```python
from build123d import *

# Parameters (mm, degrees)
SKETCH_1_R      = 1.6
SKETCH_1_R_2    = 20.5
SKETCH_1_R_3    = 12.6
EXTRUDE_1_DEPTH = 2
FILLET_1_R      = 5


with BuildPart() as part:
    # 草图1 → 凸台-拉伸1 (new body)
    # profile 1 of 2: a face of its own
    with BuildSketch(Plane(origin=(0, 0, 0), x_dir=(1, 0, 0), z_dir=(0, 1, 0))):
        with BuildLine():
            Line((-20.5, 39.5), (-20.5, 0))
            ThreePointArc((-20.5, 0), (0, 20.5), (20.5, 0))
            Line((20.5, 0), (20.5, 39.5))
            Line((20.5, 39.5), (-20.5, 39.5))
        make_face()
        with Locations(Location((-10, 32, 0), (0, 0, 270))):
            Circle(SKETCH_1_R, mode=Mode.SUBTRACT)
        with Locations(Location((10, 32, 0), (0, 0, 270))):
            Circle(SKETCH_1_R, mode=Mode.SUBTRACT)
    # profile 2 of 2: a face of its own
    with BuildSketch(Plane(origin=(0, 0, 0), x_dir=(1, 0, 0), z_dir=(0, 1, 0))):
        Circle(SKETCH_1_R_2)
        with Locations(Location((11.66726189, -11.66726189, 0), (0, 0, 270))):
            Circle(SKETCH_1_R, mode=Mode.SUBTRACT)
        with Locations(Location((11.66726189, 11.66726189, 0), (0, 0, 270))):
            Circle(SKETCH_1_R, mode=Mode.SUBTRACT)
        with Locations(Location((-11.66726189, 11.66726189, 0), (0, 0, 270))):
            Circle(SKETCH_1_R, mode=Mode.SUBTRACT)
        with Locations(Location((-11.66726189, -11.66726189, 0), (0, 0, 270))):
            Circle(SKETCH_1_R, mode=Mode.SUBTRACT)
        with Locations(Location((0, 0, 0), (0, 0, 270))):
            Circle(SKETCH_1_R_3, mode=Mode.SUBTRACT)
    extrude(amount=EXTRUDE_1_DEPTH)

    # 圆角1
    fillet_1_edges = [part.edges().sort_by_distance(p)[0] for p in [
        (-20.5, 1, -39.5),
        (20.5, 1, -39.5),
    ]]
    fillet(fillet_1_edges, radius=FILLET_1_R)


solid = part.part
```
Geometry: final body of the model. Coordinates: model frame, mm. Coordinates: 2 decimals unless noted, no trailing zeros. Order: outer loops, then holes, each group sorted by start corner. A loop starts at its lowest first (then second) coordinate and runs counter-clockwise, first axis right, second up. Notation, with made-up numbers: (22, 17) -> (81, 17) arc R21 cw to (81, 32) -> close; hole circle Ø9 at (85.5, -32.5). An arc over 180 degrees is marked (long way). Use CSV: the item, a comma, the result in double quotes.
1) Section D-D on z = -3. Output: boundary loops of the cut face in (x, y), then the cut area to 3 significant figures.
Findings:
outline,"(-20.5, 0) -> (-12.24, 0) -> (-12.24, 2) -> (-20.5, 2) -> close; (12.24, 0) -> (20.5, 0) -> (20.5, 2) -> (12.24, 2) -> close"
area,"33.0 mm^2"
2) Mould query, pull axis X, two halves, no side actions, for faces 1 (the cylindrical face through (9.03, 0.99, -33.27)), 2 (the flat face through (0, 1, -39.5)), 3 (the flat face through (20.5, 1, -17)). Classes: +X half, -X half, draft (parallel to the pull), parting line (faces both ways), or undercut.
Findings:
face 1,"undercut"
face 2,"draft"
face 3,"+X half"
3) Line query: line 1 (X direction, y = 0.4, z = -32); line 2 (X direction, y = 1.35, z = -13); line 3 (X direction, y = 0.85, z = 11). Output: solid intervals per line, ascending.
Findings:
line 1,"x = -20.5 to -11.6, -8.4 to 8.4, 11.6 to 20.5"
line 2,"x = -20.5 to -12.55, -10.78 to 10.78, 12.55 to 20.5"
line 3,"x = -17.3 to -13.12, -10.21 to -6.14, 6.14 to 10.21, 13.12 to 17.3"
4) Pin query (flat end, axial travel): pin 1 Ø1.9 at (x, z) = (10, -32) entering from -Y. Return the tip coordinate at first contact, or that it passes through.
Findings:
pin 1,"passes through"
5) Section C-C on x = -11. Output: boundary loops of the cut face in (y, z).
Findings:
outline,"(0, -39.5) -> (2, -39.5) -> (2, -33.25) -> (0, -33.25) -> close; (0, -30.75) -> (2, -30.75) -> (2, -13.12) -> (0, -13.12) -> close; (0, -10.21) -> (2, -10.21) -> (2, -6.14) -> (0, -6.14) -> close; (0, 6.14) -> (2, 6.14) -> (2, 10.21) -> (0, 10.21) -> close; (0, 13.12) -> (2, 13.12) -> (2, 17.3) -> (0, 17.3) -> close"
6) Section A-A on z = -32. Output: boundary loops of the cut face in (x, y).
Findings:
outline,"(-20.5, 0) -> (-11.6, 0) -> (-11.6, 2) -> (-20.5, 2) -> close; (-8.4, 0) -> (8.4, 0) -> (8.4, 2) -> (-8.4, 2) -> close; (11.6, 0) -> (20.5, 0) -> (20.5, 2) -> (11.6, 2) -> close"
7) Section B-B on x = 0. Output: boundary loops of the cut face in (y, z), then the cut area to 3 significant figures.
Findings:
outline,"(0, -39.5) -> (2, -39.5) -> (2, -12.6) -> (0, -12.6) -> close; (0, 12.6) -> (2, 12.6) -> (2, 20.5) -> (0, 20.5) -> close"
area,"69.6 mm^2"
